Source: CAD feature listing. Evaluate the final solid. Frame: model axes, mm. A direction names the side the tool comes from. Round coordinates to 2 decimals unless told otherwise and drop trailing zeros. Loops run counter-clockwise (first coordinate to the right, second up) from the corner with the lowest first, then second, coordinate; pieces in that order, holes last.
Item 1: Section query D-D on y = 2.5. Return loops of the section in (x, z), then the cut area to 3 significant figures.
Item 2: First-contact query: P1, Ø8, axis at x = 10.5, y = 15, coming from the +Z side; P2, Ø3, axis at y = 15, z = 6, coming from the +X side; P3, Ø3.5, axis at y = -15, z = 3.5, coming from the -X side; P4, Ø1.5, axis at x = 10.5, z = 4.5, coming from the -Y side. Flat tips, straight axial feed; report the tip coordinate or a pass-through.
Item 3: Pull-direction query (Y, two-part tool) for faces 5 (the flat face through (0, -5.81, 3)), 6 (the cylindrical face through (-3.5, -16.5, 3.6)), 7 (the flat face through (2, 20, 4)); classes: released by +Y, released by -Y, zero draft, split by the parting line, or undercut.
Item 4: Ray query, L1, parallel to Y at x = 1.25, z = 4; L2, parallel to Y at x = 3.25, z = 1; L3, parallel to X at y = 2, z = 1. Return the intervals inside material, ascending.
Item 5: Access query for faces 1 (the flat face through (-0.5, -16, 3)), 2 (the cylindrical face through (-3.5, 16.5, 3.6)), 3 (the flat face through (5.008, 2.946, 3.451)), 4 (the flat face through (-0.5, 16, 3)). Directions: +Z, -Z, +X, -X, +Y, -Y. A direction counts if a zero-diameter tool reaches every point of the face in a straight line with its end or side. Return the directions, or none.
Item 6: Section query B-B on x = 0. Return loops of the section in (y, z), then the cut area to 3 significant figures.
Item 7: Section query A-A on y = -13.5. Return loops of the section in (x, z).
Item 8: Section query C-C on z = 4. Return loops of the section in (x, y).
```python
from build123d import *

# Parameters (mm, degrees)
F1_DEPTH = 7
F3_DEPTH = 7


# Not quite as in the source:
# - a pattern or mirror of a feature is missing from the dataset's text; its kind, count and spacing are read off the source's solid


with BuildPart() as f1:
    # F0 (on Top) → F1 (new body)
    with BuildSketch(Plane.XY):
        with BuildLine():
            Line((3.6400549446, 13), (-3.6400549446, 13))
            ThreePointArc((-3.6400549446, 13), (-13.5, 0), (-3.6400549446, -13))
            Line((-3.6400549446, -13), (3.6400549446, -13))
            ThreePointArc((3.6400549446, -13), (13.5, 0), (3.6400549446, 13))
        make_face()
        Polygon((-6.7091866291, 0), (-3.3545933146, 5.8103260596), (3.3545933146, 5.8103260596), (6.7091866291, 0), (3.3545933146, -5.8103260596), (-3.3545933146, -5.8103260596), align=None, mode=Mode.SUBTRACT)
    extrude(amount=F1_DEPTH)

    # F2 (on face) → F3 (join)
    with BuildSketch(Plane.XZ.offset(13)):
        with BuildLine():
            Line((-0.5, 0.0358983849), (-0.5, 6.9641016151))
            ThreePointArc((-0.5, 6.9641016151), (-3.5, 3.5), (-0.5, 0.0358983849))
        make_face()
        with BuildLine():
            ThreePointArc((0.5, 0.0358983849), (2.6457513111, 1.2087121525), (3.5, 3.5))
            ThreePointArc((3.5, 3.5), (2.6457513111, 5.7912878475), (0.5, 6.9641016151))
            Line((0.5, 6.9641016151), (0.5, 0.0358983849))
        make_face()
    f3 = extrude(amount=F3_DEPTH)

    # F3_copies: F3 across plane
    add(f3.mirror(Plane.ZX))


solid = f1.part
```
Data:
1. outline: (-13.27, 0) - (-5.27, 0) - (-5.27, 7) - (-13.27, 7) - close; (5.27, 0) - (13.27, 0) - (13.27, 7) - (5.27, 7) - close
1. area: 112 mm2
2. P1: passes through
2. P2: stops at x = 3.35
2. P3: stops at x = -3.5
2. P4: stops at y = -9.34
3. face 5: undercut
3. face 6: zero draft
3. face 7: released by +Y
4. L1: y = -20 to -5.81, 5.81 to 20
4. L2: y = -13 to -5.81, 5.81 to 13
4. L3: x = -13.35 to -5.55, 5.55 to 13.35
5. face 1: +Z, -Z, -Y
5. face 2: -X, +Y
5. face 3: +Z, -Z
5. face 4: +Z, -Z, +Y
6. outline: (-13, 0) - (-5.81, 0) - (-5.81, 7) - (-13, 7) - close; (5.81, 0) - (13, 0) - (13, 7) - (5.81, 7) - close
6. area: 101 mm2
7. outline: (-0.5, 0.04) - (-0.5, 6.96) arc R3.5 ccw to start; (0.5, 0.04) arc R3.5 ccw to (0.5, 6.96) - close
8. outline: (-3.64, -13) - (-3.46, -13) - (-3.46, -20) - (-0.5, -20) - (-0.5, -13) - (0.5, -13) - (0.5, -20) - (3.46, -20) - (3.46, -13) - (3.64, -13) arc R13.5 ccw to (3.64, 13) - (3.46, 13) - (3.46, 20) - (0.5, 20) - (0.5, 13) - (-0.5, 13) - (-0.5, 20) - (-3.46, 20) - (-3.46, 13) - (-3.64, 13) arc R13.5 ccw to start; hole (-6.71, 0) - (-3.35, -5.81) - (3.35, -5.81) - (6.71, 0) - (3.35, 5.81) - (-3.35, 5.81) - close
